```python
from build123d import *

# Parameters (mm, degrees)
BOSS_EXTRUDE1_DEPTH      = 1
SKETCH1_3_W              = 2.5
SKETCH1_3_H              = 12
BOSS_EXTRUDE2_DEPTH      = 15.5
F_3_0_3_DIAMETER_HOLE1_D = 3
SKETCH6_W                = 6.5
SKETCH6_H                = 2
BOSS_EXTRUDE3_DEPTH      = 24
SKETCH6_4_W              = 7
SKETCH6_4_H              = 8
CUT_EXTRUDE1_DEPTH       = 26.85
SKETCH8_W                = 7
SKETCH8_H                = 19.5
CUT_EXTRUDE2_DEPTH       = 8.5
CUT_EXTRUDE3_DEPTH       = 0.3


with BuildPart() as part:
    # Sketch1 → Boss-Extrude1 (new body)
    with BuildSketch(Plane(origin=(0, 0, 0), x_dir=(1, 0, 0), z_dir=(0, 1, 0))):
        Polygon((-21.75, 31.85), (0, 31.85), (0, 76.35), (-26.25, 76.35), (-26.25, 53.35), (-26.25, 41.35), (-26.25, 31.85), align=None)
        Polygon((0, 76.35), (0, 31.85), (21.75, 31.85), (26.25, 31.85), (26.25, 76.35), align=None)
    extrude(amount=BOSS_EXTRUDE1_DEPTH)

    # Sketch1_3 → Boss-Extrude2 (add)
    with BuildSketch(Plane(origin=(0, 0, 0), x_dir=(1, 0, 0), z_dir=(0, 1, 0))):
        Polygon((-26.25, 31.85), (-26.25, 41.35), (-28.75, 41.35), (-28.75, 0), (-21.75, 0), (-21.75, 31.85), align=None)
        Polygon((-26.25, 76.35), (-28.75, 76.35), (-28.75, 74.35), (-28.75, 68.35), (-28.75, 53.35), (-26.25, 53.35), align=None)
        Polygon((28.75, 76.35), (26.25, 76.35), (26.25, 31.85), (21.75, 31.85), (21.75, 0), (28.75, 0), (28.75, 68.35), (28.75, 74.35), align=None)
        with Locations((-27.5, 47.35)):
            Rectangle(SKETCH1_3_W, SKETCH1_3_H)
    extrude(amount=BOSS_EXTRUDE2_DEPTH)

    # 3.0 _3_ Diameter Hole1 (through all)
    with Locations(Plane(origin=(0, 0, 0), x_dir=(-1, 0, 0), z_dir=(0, -1, 0))):
        with Locations((-22.85, 73.45), (22.85, 73.45), (26, 29.35), (22.85, 35.4), (-22.85, 35.4), (-26, 29.35), (-26, 3), (26, 3), (-30.25, 71.35), (30.25, 71.35)):
            Hole(F_3_0_3_DIAMETER_HOLE1_D / 2)

    # Sketch6 → Boss-Extrude3 (add)
    with BuildSketch(Plane.XY):
        Polygon((20.25, 10.5), (21.75, 10.5), (21.75, 12.5), (15.25, 12.5), (15.25, 10.5), align=None)
        with Locations((-18.5, 11.5)):
            Rectangle(SKETCH6_W, SKETCH6_H)
    extrude(amount=-BOSS_EXTRUDE3_DEPTH)

    # Sketch6_4 → Cut-Extrude1 (cut)
    with BuildSketch(Plane.XY):
        with Locations((-25.25, 4)):
            Rectangle(SKETCH6_4_W, SKETCH6_4_H)
        with Locations((25.25, 4)):
            Rectangle(SKETCH6_4_W, SKETCH6_4_H)
    extrude(amount=-CUT_EXTRUDE1_DEPTH, mode=Mode.SUBTRACT)

    # Sketch8 → Cut-Extrude2 (cut)
    with BuildSketch(Plane.XZ):
        with Locations((-25.25, -51.6)):
            Rectangle(SKETCH8_W, SKETCH8_H)
        with Locations((25.25, -51.6)):
            Rectangle(SKETCH8_W, SKETCH8_H)
    extrude(amount=-CUT_EXTRUDE2_DEPTH, mode=Mode.SUBTRACT)

    # Sketch9 → Cut-Extrude3 (cut)
    with BuildSketch(Plane.XZ):
        Polygon((-10.502040481, -57.1), (4.24240096, -39.528258941), (2.025663817, -52.1), (10.502040481, -52.1), (-4.24240096, -69.671741059), (-2.025663817, -57.1), align=None)
        Polygon((-3.425965173, -67.920888862), (-1.429787021, -56.6), (-9.429787021, -56.6), (3.425965173, -41.279111138), (1.429787021, -52.6), (9.429787021, -52.6), align=None, mode=Mode.SUBTRACT)
    extrude(amount=-CUT_EXTRUDE3_DEPTH, mode=Mode.SUBTRACT)


solid = part.part
```
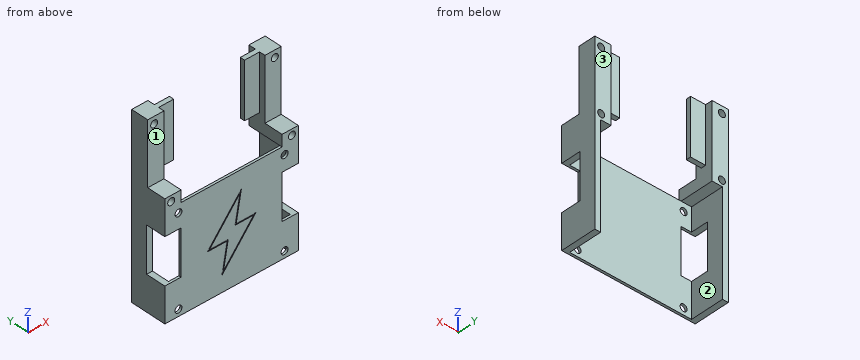
Read the model definition and answer for the solid it produces. Units are mm, in the model's axes. Face numbers are marked on the shaded views. A direction names the side the tool comes from. Coordinates: 2 decimals unless noted, no trailing zeros. Order: outer loops, then holes, each group sorted by start corner. A loop starts at its lowest first (then second) coordinate and runs counter-clockwise, first axis right, second up. Notation, with made-up numbers: (1.5, -22.75) - (40.5, -22.75) arc R17 cw to (40.5, 4.25) - close; hole circle Ø2 at (27, -18.5). An arc over 180 degrees is marked (long way). Answer as a JSON object with one key per item and string values. Group by question number.
Item 1: Section B-B (y = 11.5) is taken. Give the vertices of the cut face in (x, z), plus the area to 3 significant figures.
Item 2: Consider probe 1 along X at (y, z) = (0.75, -73.45); probe 2 along Z at (x, y) = (-26, 10.5); probe 3 along Z at (x, y) = (-22.85, 0.7). Determine where each line is inside the solid, lowest interval first. Write a range as from..to.
Item 3: Section D-D (y = 3.25) is taken. Give the vertices of the cut face in (x, z).
Item 4: Section C-C (x = -22.85) is taken. Give the vertices of the cut face in (y, z), plus the area to 3 significant figures.
Item 5: Flat-ended cylindrical pins translate along their axes: P1, Ø7, axis at x = -19.5, z = -17.5, coming from the -Y side; P2, Ø4, axis at x = -22.85, z = -73.45, coming from the +Y side; P3, Ø2, axis at x = 23, y = 12.5, coming from the -Z side. Find the tip coordinate at first contact, or state that the pin passes through.
Item 6: A tool of negligible diameter and unlimited length cuts with its end or side. For the marked faces 1, 2 and 3, from which of +Z, -Z, +X, -X, +Y, -Y can it reach the whole face along a straight path? Write none if from no direction.
Item 7: Section A-A (z = -29.35) is taken. Give the vertices of the cut face in (x, y), plus the area to 3 significant figures.
Results are:
{
 "1": {"outline": "(-28.75, -76.35) - (-26.25, -76.35) - (-26.25, -31.85) - (-21.75, -31.85) - (-21.75, -24) - (-15.25, -24) - (-15.25, 0) - (-28.75, 0) - close; (15.25, -24) - (21.75, -24) - (21.75, -31.85) - (26.25, -31.85) - (26.25, -76.35) - (28.75, -76.35) - (28.75, 0) - (15.25, 0) - close; hole circle Ø3 at (-26, -29.35); hole circle Ø3 at (-26, -3); hole circle Ø3 at (26, -29.35); hole circle Ø3 at (26, -3)", "area": "952 mm^2"},
 "2": {"probe 1": "x = -28.75..-24.35, -21.35..21.35, 24.35..28.75", "probe 2": "z = -31.85..-30.85, -27.85..-4.5, -1.5..0", "probe 3": "z = -76.35..-74.95, -71.95..-61.35, -41.85..-36.9, -33.9..-26.85"},
 "3": {"outline": "(-28.75, -76.35) - (-26.25, -76.35) - (-26.25, -61.35) - (-28.75, -61.35) - close; (-28.75, -41.85) - (-26.25, -41.85) - (-26.25, -31.85) - (-21.75, -31.85) - (-21.75, -26.85) - (-28.75, -26.85) - close; (21.75, -31.85) - (26.25, -31.85) - (26.25, -41.85) - (28.75, -41.85) - (28.75, -26.85) - (21.75, -26.85) - close; (26.25, -76.35) - (28.75, -76.35) - (28.75, -61.35) - (26.25, -61.35) - close; hole circle Ø3 at (-26, -29.35); hole circle Ø3 at (26, -29.35)"},
 "4": {"outline": "(0, -76.35) - (1, -76.35) - (1, -74.95) - (0, -74.95) - close; (0, -71.95) - (1, -71.95) - (1, -61.35) - (0, -61.35) - close; (0, -41.85) - (1, -41.85) - (1, -36.9) - (0, -36.9) - close; (0, -33.9) - (1, -33.9) - (1, -31.85) - (15.5, -31.85) - (15.5, 0) - (8, 0) - (8, -26.85) - (0, -26.85) - close", "area": "298 mm^2"},
 "5": {"P1": "stops at y = 8", "P2": "stops at y = 1", "P3": "stops at z = -31.85"},
 "6": {"face 1": "+Z, +X, -X, -Y", "face 2": "-Z, +Y", "face 3": "+Z, -Z, +X, -X, +Y"},
 "7": {"outline": "(-28.75, 0) - (-27.5, 0) - (-27.5, 15.5) - (-28.75, 15.5) - close; (-24.5, 0) - (-21.75, 0) - (-21.75, 15.5) - (-24.5, 15.5) - close; (21.75, 0) - (24.5, 0) - (24.5, 15.5) - (21.75, 15.5) - close; (27.5, 0) - (28.75, 0) - (28.75, 15.5) - (27.5, 15.5) - close", "area": "124 mm^2"}
}
